Read the model definition and answer for the solid it produces. Units are mm, in the model's axes. A direction names the side the tool comes from. Coordinates: 2 decimals unless noted, no trailing zeros. Write each loop counter-clockwise with the first axis right and the second up, starting at its lowest first coordinate (ties: lowest second). Pieces come first, ordered by that corner, then holes.
from build123d import *

# Parameters (mm, degrees)
SKETCH_R     = 9
PAD_DEPTH    = 65
SKETCH001_R  = 3
PAD001_DEPTH = 2.25
FILLET_R     = 0.75
FILLET001_R  = 1
SKETCH002_R  = 5
PAD002_DEPTH = 0.25
SKETCH003_R  = 5
PAD003_DEPTH = 0.25


with BuildPart() as part:
    # Sketch → Pad (new body)
    with BuildSketch(Plane.XY):
        Circle(SKETCH_R)
    extrude(amount=PAD_DEPTH)

    # Sketch001 (on Face3 of Pad) → Pad001 (join)
    with BuildSketch(Plane.XY.offset(65)):
        Circle(SKETCH001_R)
    extrude(amount=PAD001_DEPTH)

    # Fillet
    fillet_edges = [part.edges().sort_by_distance(p)[0] for p in [
        (-3, 0, 67.25),
    ]]
    fillet(fillet_edges, radius=FILLET_R)

    # Fillet001
    fillet001_edges = [part.edges().sort_by_distance(p)[0] for p in [
        (-9, 0, 0),
        (-9, 0, 65),
    ]]
    fillet(fillet001_edges, radius=FILLET001_R)

    # Sketch002 (on Face1 of Fillet001) → Pad002 (join)
    with BuildSketch(Plane.XY.offset(65)):
        Circle(SKETCH002_R)
    extrude(amount=PAD002_DEPTH)

    # Sketch003 (on Face8 of Pad002) → Pad003 (join)
    with BuildSketch(Plane(origin=(0, 0, 0), x_dir=(1, 0, 0), z_dir=(0, 0, -1))):
        Circle(SKETCH003_R)
    extrude(amount=PAD003_DEPTH)


solid = part.part
Item 1: Given pin 1 (6 mm diameter, centred on x = 3, z = 49.5, fed in from -Y); pin 2 (5 mm diameter, centred on y = 6, z = 8.5, fed in from +X); pin 3 (1.5 mm diameter, centred on x = 6, z = 16.5, fed in from -Y); pin 4 (3 mm diameter, centred on x = 6.5, y = 3, fed in from -Z), each flat-ended and moving along its own axis, determine where each tip first touches the part or whether it passes through.
Item 2: For faces 1 (the flat face through (-0.1, -5.2, 0)), 2 (the flat face through (0, 0, 67.25)), 3 (the cylindrical face through (-3, 0, 66)), determine the directions among +Z, -Z, +X, -X, +Y, -Y from which every point of the face is accessible in a straight line to the end or side of a thin tool.
Item 3: Find the intervals of material crossed by probe 1 along Z at (x, y) = (5, 0.75); probe 2 along Y at (x, z) = (-0.5, 3.5); probe 3 along Y at (x, z) = (1.5, 64), in increasing order.
Item 4: The part is cut by section C-C (z = 4). Give the vertices of the cut face in (x, y), and give its area (3 significant figures).
Item 5: The part is cut by section A-A (x = 0). Give the vertices of the cut face in (y, z).
Answer:
1. pin 1: stops at y = -9
1. pin 2: stops at x = 8.29
1. pin 3: stops at y = -7.31
1. pin 4: stops at z = 0
2. face 1: -Z
2. face 2: +Z, +X, -X, +Y, -Y
2. face 3: +Z
3. probe 1: z = 0 to 65
3. probe 2: y = -8.99 to 8.99
3. probe 3: y = -8.87 to 8.87
4. outline: circle Ø18 at (0, 0)
4. area: 254 mm2
5. outline: (-9, 1) arc R1 ccw to (-8, 0) - (-5, 0) - (-5, -0.25) - (5, -0.25) - (5, 0) - (8, 0) arc R1 ccw to (9, 1) - (9, 64) arc R1 ccw to (8, 65) - (5, 65) - (5, 65.25) - (3, 65.25) - (3, 66.5) arc R0.75 ccw to (2.25, 67.25) - (-2.25, 67.25) arc R0.75 ccw to (-3, 66.5) - (-3, 65.25) - (-5, 65.25) - (-5, 65) - (-8, 65) arc R1 ccw to (-9, 64) - close
